Read the model definition and answer for the solid it produces. Units are mm, in the model's axes. A direction names the side the tool comes from. Coordinates: 2 decimals unless noted, no trailing zeros. Loops run counter-clockwise (first coordinate to the right, second up) from the corner with the lowest first, then second, coordinate; pieces in that order, holes last. Notation, with made-up numbers: (57.25, 5.5) -> (70.25, 5.5) arc R25 ccw to (70.25, 21.5) -> close; hole circle Ø11 at (9, 38.25). An arc over 180 degrees is marked (long way). Answer as a JSON object with one key per item and string values. Group by question number.
Q1. For faces 1 (the flat face through (0, 0, 0)), 2 (the cylindrical face through (4.82, -9.27, 13.73)), determine the directions among +Z, -Z, +X, -X, +Y, -Y from which every point of the face is accessible in a straight line to the end or side of a thin tool.
Q2. Straight lines are drawn through the part: line 1 along Y through (x, z) = (0, 14.1); line 2 along Z through (x, y) = (-13.5, -3.25); line 3 along Y through (x, z) = (-7, 13.75). For each, find the intervals that lie inside material, in ascending order. Write a range as [from, to].
Q3. The part is cut by section D-D on y = -5. Write down the section's boundary in (x, z).
Q4. Determine the mould class of faces 3 (the flat face through (-14, 0, 12.5)), 4 (the flat face through (4.5, 0.1, 12.5)), 5 (the flat face through (0, -15, 6)), 6 (the cylindrical face through (3.67, -1.52, 13.73)) for opening direction Y: released by +Y, released by -Y, zero draft, split by the parting line, or undercut.
Q5. The part is cut by section A-A on z = 13.5. Write down the section's boundary in (x, y), and give its area (3 significant figures).
Q6. This flat-tipped pin is pushed along its axis until it touches: P1, Ø1, axis at x = 10.5, y = -12, coming from the +Z side. Where does it stop, or does it pass through?
Q7. The part is cut by section B-B on x = 0. Write down the section's boundary in (y, z), and give its area (3 significant figures).
from build123d import *

# Parameters (mm, degrees)
F0_W     = 30
F0_H     = 30
F1_DEPTH = 12.5
F3_R     = 13.460872
F3_R_2   = 10.447171
F4_DEPTH = 2.5
F2_R     = 3.97173
F5_DEPTH = 2.5


with BuildPart() as f1:
    # F0 (on Top) → F1 (new body)
    with BuildSketch(Plane.XY):
        Rectangle(F0_W, F0_H)
    extrude(amount=F1_DEPTH)

    # F3 (on face) → F4 (join)
    with BuildSketch(Plane.XY.offset(12.5)):
        Circle(F3_R)
        Circle(F3_R_2, mode=Mode.SUBTRACT)
    extrude(amount=F4_DEPTH)

    # F2 (on face) → F5 (join)
    with BuildSketch(Plane.XY.offset(12.5)):
        Circle(F2_R)
    extrude(amount=F5_DEPTH)


solid = f1.part
Final values:
{
 "1": {"face 1": "-Z, +X, -X, +Y, -Y", "face 2": "+Z"},
 "2": {"line 1": "y = [-13.46, -10.45], [-3.97, 3.97], [10.45, 13.46]", "line 2": "z = [0, 12.5]", "line 3": "y = [-11.5, -7.76], [7.76, 11.5]"},
 "3": {"outline": "(-15, 0) -> (15, 0) -> (15, 12.5) -> (12.5, 12.5) -> (12.5, 15) -> (9.17, 15) -> (9.17, 12.5) -> (-9.17, 12.5) -> (-9.17, 15) -> (-12.5, 15) -> (-12.5, 12.5) -> (-15, 12.5) -> close"},
 "4": {"face 3": "zero draft", "face 4": "undercut", "face 5": "released by -Y", "face 6": "undercut"},
 "5": {"outline": "circle Ø26.92 at (0, 0); circle Ø7.94 at (0, 0); hole circle Ø20.89 at (0, 0)", "area": "276 mm2"},
 "6": {"P1": "stops at z = 12.5"},
 "7": {"outline": "(-15, 0) -> (15, 0) -> (15, 12.5) -> (13.46, 12.5) -> (13.46, 15) -> (10.45, 15) -> (10.45, 12.5) -> (3.97, 12.5) -> (3.97, 15) -> (-3.97, 15) -> (-3.97, 12.5) -> (-10.45, 12.5) -> (-10.45, 15) -> (-13.46, 15) -> (-13.46, 12.5) -> (-15, 12.5) -> close", "area": "410 mm2"}
}
